Source: CAD feature listing. Evaluate the final solid. Frame: model axes, mm. Give positions to 0.01 mm unless a question says otherwise; leave off trailing zeros. Loops run counter-clockwise (first coordinate to the right, second up) from the corner with the lowest first, then second, coordinate; pieces in that order, holes last.
```python
from build123d import *

# Parameters (mm, degrees)
BOSS_EXTRUDE1_DEPTH = 3.175
SKETCH2_R           = 2.032
CUT_EXTRUDE1_DEPTH  = 101.626437428
FILLET1_R           = 4.445


with BuildPart() as part:
    # Sketch1 → Boss-Extrude1 (new body)
    with BuildSketch(Plane(origin=(0, 0, 0), x_dir=(1, 0, 0), z_dir=(0, 1, 0))):
        with BuildLine():
            Line((53.764572514, 19.37764801), (89.607620856, 32.296080017))
            ThreePointArc((89.607620856, 32.296080017), (95.25, 0), (89.607620856, -32.296080017))
            Line((89.607620856, -32.296080017), (53.764572514, -19.37764801))
            ThreePointArc((53.764572514, -19.37764801), (57.15, 0), (53.764572514, 19.37764801))
        make_face()
    extrude(amount=BOSS_EXTRUDE1_DEPTH)

    # Sketch2 → Cut-Extrude1 (cut, through all)
    with BuildSketch(Plane(origin=(0, 3.175, 0), x_dir=(1, 0, 0), z_dir=(0, 1, 0))):
        with Locations(Location((87.702620856, 25.946080017, 0), (0, 0, 270))):
            Circle(SKETCH2_R)
    extrude(amount=-CUT_EXTRUDE1_DEPTH, mode=Mode.SUBTRACT)

    # Fillet1
    fillet1_edges = [part.edges().sort_by_distance(p)[0] for p in [
        (53.764572514, 1.5875, -19.37764801),
        (89.607620856, 1.5875, -32.296080017),
        (89.607620856, 1.5875, 32.296080017),
        (53.764572514, 1.5875, 19.37764801),
    ]]
    fillet(fillet1_edges, radius=FILLET1_R)


solid = part.part
```
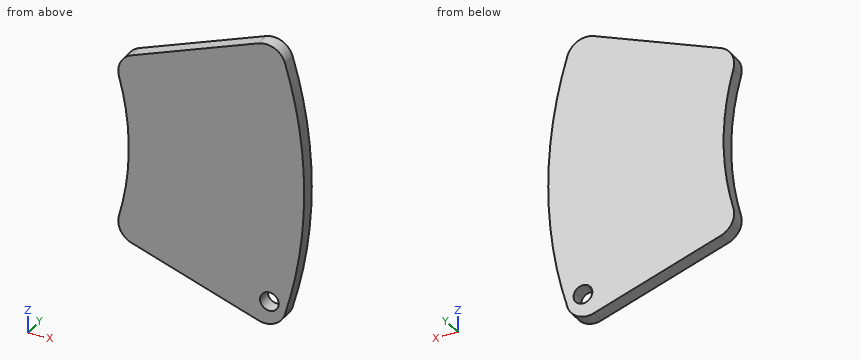
(1) First-contact query: pin 1 (1.5 mm diameter, centred on y = 3, z = -19.5, fed in from -X). Flat tip, straight axial feed; report the tip coordinate or a pass-through.
A:
pin 1: stops at x = 55.39
(2) Ray query, line 1 along Z through (x, y) = (89.5, 2.3); line 2 along Z through (x, y) = (87, 1.3); line 3 along X through (y, z) = (0.9, 9.5). Return the intervals inside material, ascending.
A:
line 1: z = -30.12 to -26.89, -25 to 30.12
line 2: z = -31.01 to -27.85, -24.04 to 31.01
line 3: x = 56.35 to 94.78
(3) Section C-C, the plane z = -9. Return the cut outline in (x, y) (3 decimals), then the cut area to 3 significant figures.
A:
outline: (56.437, 0) - (94.824, 0) - (94.824, 3.175) - (56.437, 3.175) - close
area: 122 mm2
(4) Section A-A, the plane y = 1. Return the cut outline in (x, z) (3 decimals).
A:
outline: (55.023, -15.447) arc R4.445 ccw to (57.795, -20.83) - (85.324, -30.752) arc R4.445 ccw to (91.081, -27.871) arc R95.25 ccw to (91.081, 27.871) arc R4.445 ccw to (85.324, 30.752) - (57.795, 20.83) arc R4.445 ccw to (55.023, 15.447) arc R57.15 cw to start; hole circle Ø4.064 at (87.703, -25.946)
(5) Section B-B, the plane x = 81. Return the cut outline in (y, z) (3 decimals), then the cut area to 3 significant figures.
A:
outline: (0, -29.194) - (3.175, -29.194) - (3.175, 29.194) - (0, 29.194) - close
area: 185 mm2
